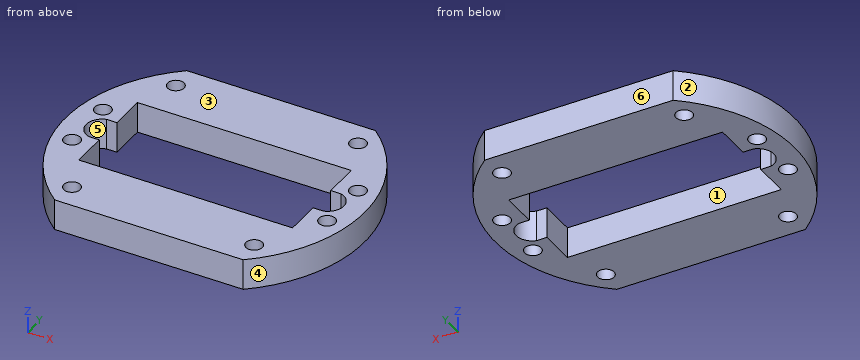
Autodesk Inventor part; units mm, degrees
ref_plane "YZ Plane" through (0, 0, 0) normal (1, 0, 0) x (0, 1, 0)
ref_plane "XZ Plane" through (0, 0, 0) normal (0, 1, 0) x (-1, 0, 0)
ref_plane "XY Plane" through (0, 0, 0) normal (0, 0, 1) x (1, 0, 0)
sketch "Эскиз1" plane through (0, 0, 0) normal (0, 0, 1) x (1, 0, 0)
  line L0 (-20.75, 10) -> (20.75, 10)
  line L1 (20.75, 10) -> (20.75, -10)
  line L2 (20.75, -10) -> (-20.75, -10)
  line L3 (-20.75, -10) -> (-20.75, 10)
  line L4 (-20.75, 10) -> (20.75, -10) construction
  line L5 (20.75, 10) -> (-20.75, -10) construction
  circle A0 centre (0, 0) radius 29
  line L6 (0, 0) -> (0, 105.5742) construction
  line L7 (0, 0) -> (104.4464, 0) construction
  circle A1 centre (0, 0) radius 25 construction
  line L8 (0, 0) -> (29.0219, 29.0219) construction
  circle A2 centre (17.6777, 17.6777) radius 1.6
  line L9 (0, 0) -> (-29.0219, 29.0219) construction
  circle A3 centre (-17.6777, 17.6777) radius 1.6
  line L10 (0, 0) -> (-29.0219, -29.0219) construction
  circle A4 centre (-17.6777, -17.6777) radius 1.6
  line L11 (0, 0) -> (29.0219, -29.0219) construction
  circle A5 centre (17.6777, -17.6777) radius 1.6
  circle A6 centre (-24.75, -5.25) radius 1.6
  circle A7 centre (-24.75, 5.25) radius 1.6
  circle A8 centre (24.75, -5.25) radius 1.6
  circle A9 centre (24.75, 5.25) radius 1.6
  line L12 (20.75, 3) -> (22.75, 3)
  line L13 (22.75, 3) -> (22.75, -3)
  line L14 (22.75, -3) -> (20.75, -3)
  line L15 (20.75, -3) -> (20.75, 3)
  line L16 (-20.75, 3) -> (-22.75, 3)
  line L17 (-22.75, 3) -> (-22.75, -3)
  line L18 (-22.75, -3) -> (-20.75, -3)
  line L19 (-20.75, -3) -> (-20.75, 3)
  line L20 (-18.2962, -22.5) -> (18.2962, -22.5)
  line L21 (-18.2962, 22.5) -> (18.2962, 22.5)
  arc A10 (22.75, -3) -> (22.75, 3) centre (21.875, 0) ccw
  arc A11 (-22.75, 3) -> (-22.75, -3) centre (-21.875, 0) ccw
  point P0 (-20.75, -3)
  point P1 (-20.75, 3)
  dimension "d18" = 50
  dimension "d0" = 41.5
  dimension "d1" = 20
  dimension "d8" = 58
  dimension "d17" = 45
  dimension "d19" = 3.2
  dimension "d22" = 360
  dimension "d24" = 3.2
  dimension "d25" = 4.75
  dimension "d26" = 4
  dimension "d29" = 4.75
  dimension "d31" = 2
  dimension "d32" = 6
  dimension "d33" = 2
  dimension "d34" = 45
extrude "Выдавливание1" add sketch "Эскиз1" along normal mid plane 6 contours A0 L20 L21
properties part number "Кронштейн_сервопривод"
Geometry: final body of the model. Coordinates: model frame, mm. Face numbers are marked on the shaded views. A direction names the side the tool comes from. Round coordinates to 2 decimals unless told otherwise and drop trailing zeros. Order: outer loops, then holes, each group sorted by start corner. A loop starts at its lowest first (then second) coordinate and runs counter-clockwise, first axis right, second up. Notation, with made-up numbers: (-16, 40.25) -> (-1, 40.25) arc R35 cw to (-1, 75.25) -> close; hole circle Ø8 at (10, -39.75). An arc over 180 degrees is marked (long way). Use CSV: the item, a comma, the result in double quotes. Start each with the question number.
1) Material intervals for line 1 along Y through (x, z) = (-12, -2.15); line 2 along Y through (x, z) = (-24.75, -1.55); line 3 along X through (y, z) = (18.5, -2.15), sorted ascending. Write a range as from..to.
2) Section D-D (y = 5.25). Return the cut outline in (x, z).
3) Draft query along Y for the marked faces 3, 4, 5 and 6. Return one class per face: +Y half, -Y half, draft (parallel to the pull), parting line (faces both ways), or undercut.
4) Section A-A (x = -9.5). Return the cut outline in (y, z), and give its area (3 significant figures).
5) First-contact query: pin 1 Ø1.8 at (y, z) = (-6, 1.5) entering from -X; pin 2 Ø2 at (x, z) = (21.5, 1.5) entering from +Y; pin 3 Ø2 at (x, z) = (21.5, 0.5) entering from -Y; pin 4 Ø2.5 at (x, y) = (17.68, 17.68) entering from -Z. Flat tips, straight axial feed; report the tip coordinate or a pass-through.
6) Section C-C (z = 0.8). State how many separate pieces and enclosed holes the cut face has, and give its area (3 significant figures).
7) Set-up query: the marked faces 1 and 2. Return all of +Z, -Z, +X, -X, +Y, -Y with unobstructed straight access to the full face (end or side cutting, diameter ignored); none if empty.
8) Section B-B (x = -17.5). Return the cut outline in (y, z), and give its area (3 significant figures).
Returned:
1,line 1,"y = -22.5..-10, 10..22.5"
1,line 2,"y = -15.11..-6.85, -3.65..-1.22, 1.22..3.65, 6.85..15.11"
1,line 3,"x = -22.33..-19.05, -16.31..16.31, 19.05..22.33"
2,outline,"(-28.52, -3) -> (-26.35, -3) -> (-26.35, 3) -> (-28.52, 3) -> close; (-23.15, -3) -> (-20.75, -3) -> (-20.75, 3) -> (-23.15, 3) -> close; (20.75, -3) -> (23.15, -3) -> (23.15, 3) -> (20.75, 3) -> close; (26.35, -3) -> (28.52, -3) -> (28.52, 3) -> (26.35, 3) -> close"
3,face 3,"draft"
3,face 4,"parting line"
3,face 5,"undercut"
3,face 6,"+Y half"
4,outline,"(-22.5, -3) -> (-10, -3) -> (-10, 3) -> (-22.5, 3) -> close; (10, -3) -> (22.5, -3) -> (22.5, 3) -> (10, 3) -> close"
4,area,"150 mm²"
5,pin 1,"stops at x = -28.55"
5,pin 2,"stops at y = 20.51"
5,pin 3,"stops at y = -20.51"
5,pin 4,"passes through"
6,separate pieces,"1"
6,enclosed holes,"9"
6,area,"1,380 mm²"
7,face 1,"+Z, -Z"
7,face 2,"+Z, -Z, -X"
8,outline,"(-22.5, -3) -> (-19.27, -3) -> (-19.27, 3) -> (-22.5, 3) -> close; (-16.09, -3) -> (-10, -3) -> (-10, 3) -> (-16.09, 3) -> close; (10, -3) -> (16.09, -3) -> (16.09, 3) -> (10, 3) -> close; (19.27, -3) -> (22.5, -3) -> (22.5, 3) -> (19.27, 3) -> close"
8,area,"112 mm²"
